from build123d import *

# Parameters (mm, degrees)
SKETCH_1_R          = 15
SKETCH_1_W          = 10.1
SKETCH_1_H          = 10.1
EXTRUDE_1_DEPTH     = 80
SKETCH1_R           = 19
SKETCH1_W           = 10.1
SKETCH1_H           = 10.1
BOSS_EXTRUDE1_DEPTH = 3
CHAMFER1_SIZE       = 1
CHAMFER1_SIZE2      = 2.747477419


with BuildPart() as part:
    # Эскиз1 → Бобышка-Вытянуть1 (new body)
    with BuildSketch(Plane(origin=(0, 0, 0), x_dir=(1, 0, 0), z_dir=(0, 1, 0))):
        Circle(SKETCH_1_R)
        Rectangle(SKETCH_1_W, SKETCH_1_H, mode=Mode.SUBTRACT)
    extrude(amount=EXTRUDE_1_DEPTH)

    # Sketch1 → Boss-Extrude1 (add)
    with BuildSketch(Plane(origin=(0, 80, 0), x_dir=(1, 0, 0), z_dir=(0, 1, 0))):
        Circle(SKETCH1_R)
        Rectangle(SKETCH1_W, SKETCH1_H, mode=Mode.SUBTRACT)
    extrude(amount=-BOSS_EXTRUDE1_DEPTH)

    # Chamfer1
    chamfer1_edges = [part.edges().sort_by_distance(p)[0] for p in [
        (0, 80, -5.05),
        (-5.05, 80, 0),
        (0, 80, 5.05),
        (5.05, 80, 0),
    ]]
    chamfer1_side = [part.faces().sort_by_distance(p)[0] for p in [
        (-18.462598846, 80, 0),
    ]]
    chamfer(chamfer1_edges, length=CHAMFER1_SIZE, length2=CHAMFER1_SIZE2, reference=chamfer1_side[0])


solid = part.part
Here's how the part is built. I have some questions about the finished solid (model axes, mm). A direction names the side the tool comes from. Give positions to 0.01 mm unless a question says otherwise; leave off trailing zeros. Write each loop counter-clockwise with the first axis right and the second up, starting at its lowest first coordinate (ties: lowest second). Pieces come first, ordered by that corner, then holes. Notation, with made-up numbers: (-10.75, -32) -> (25.25, -32) arc R21 cw to (25.25, 3) -> close; hole circle Ø6 at (38.25, 20.5). An arc over 180 degrees is marked (long way). Use one line per item in the form item = value. Start each with the question number.
1. Thinking about a two-plate mould opening in X: for faces 1 (the face through (5.543, 78.607, 0.085)), 2 (the face through (-14.985, 37.961, -0.66)), 3 (the face through (6, 0, 0)), 4 (the face through (0, 38, 5.05)), which applies, +X half, -X half, draft (parallel to the pull), parting line (faces both ways), or undercut?
2. Imagine slicing it at A-A on z = 0. List the corners of the cut face in (x, y) for me.
3. If I drill on L1, parallel to Z at x = 0.5, y = 36; L2, parallel to X at y = 9.5, z = 3; L3, parallel to Y at x = -1, z = 16, over which ranges is the centre line in solid material (lowest first)?
4. Imagine slicing it at D-D on x = -9.5. List the corners of the cut face in (y, z) for me.
5. Imagine slicing it at B-B on x = 0. List the corners of the cut face in (y, z) for me.
6. On a 3-axis mill with a long thin cutter (end or side, diameter ignored), from which of +Z, -Z, +X, -X, +Y, -Y can I reach the whole of each face in a straight line? I mean faces 5 (the face through (14, 77, -6)), 6 (the face through (8, 80, 0)), 7 (the face through (-0.085, 78.607, -5.543)), 8 (the face through (5.05, 38, 0)). Say none if no direction works.
7. Will these pins go through, and if not, where does the flat tip stop? pin 1 Ø1.5 at (y, z) = (41.5, -8.5) entering from -X; pin 2 Ø2 at (x, z) = (-14, -5) entering from -Y; pin 3 Ø11 at (x, y) = (1.5, 33) entering from -Z; pin 4 Ø10 at (y, z) = (44, -13) entering from +X.
8. Imagine slicing it at C-C on y = 49. List the corners of the cut face in (x, z) for me.
Entries:
q1.face_1 = undercut
q1.face_2 = parting line
q1.face_3 = draft
q1.face_4 = undercut
q2.outline = (-19, 77) -> (-15, 77) -> (-15, 0) -> (-5.05, 0) -> (-5.05, 77.25) -> (-6.05, 80) -> (-19, 80) -> close; (5.05, 0) -> (15, 0) -> (15, 77) -> (19, 77) -> (19, 80) -> (6.05, 80) -> (5.05, 77.25) -> close
q3.L1 = -14.99 to -5.05, 5.05 to 14.99
q3.L2 = -14.7 to -5.05, 5.05 to 14.7
q3.L3 = 77 to 80
q4.outline = (0, -11.61) -> (77, -11.61) -> (77, -16.45) -> (80, -16.45) -> (80, 16.45) -> (77, 16.45) -> (77, 11.61) -> (0, 11.61) -> close
q5.outline = (0, -15) -> (77, -15) -> (77, -19) -> (80, -19) -> (80, -6.05) -> (77.25, -5.05) -> (0, -5.05) -> close; (0, 5.05) -> (77.25, 5.05) -> (80, 6.05) -> (80, 19) -> (77, 19) -> (77, 15) -> (0, 15) -> close
q6.face_5 = -Y
q6.face_6 = +Z, -Z, +X, -X, +Y
q6.face_7 = +Y
q6.face_8 = +Y, -Y
q7.pin_1 = -12.84
q7.pin_2 = 0
q7.pin_3 = -15
q7.pin_4 = 12.69
q8.outline = circle Ø30 at (0, 0); hole (-5.05, -5.05) -> (5.05, -5.05) -> (5.05, 5.05) -> (-5.05, 5.05) -> close
